Verification items for the finished model (mm, model axes). A direction names the side the tool comes from. Coordinates: 2 decimals unless noted, no trailing zeros. Order: outer loops, then holes, each group sorted by start corner. A loop starts at its lowest first (then second) coordinate and runs counter-clockwise, first axis right, second up. Notation, with made-up numbers: M -39.5,23.5 L -24.5,23.5 A16 ccw -24.5,48.5 Z; hole C 15.25,-26.5 d4. An arc over 180 degrees is marked long. Use one line per item in the form item = value. Start each with the question number.
```python
from build123d import *

# Parameters (mm, degrees)
CUBE002_W     = 38
CUBE002_H     = 3
CUBE002_DEPTH = 43.8
CUBE001_W     = 38
CUBE001_H     = 19
CUBE001_DEPTH = 43.8
SKETCH002_W   = 38
SKETCH002_H   = 43.8
PAD002_DEPTH  = 17
SKETCH003_R   = 1.2
PAD003_DEPTH  = 9
SKETCH004_W   = 38
SKETCH004_H   = 43.8
SKETCH004_W_2 = 34
SKETCH004_H_2 = 39.8
PAD004_DEPTH  = 9


with BuildPart() as cube002:
    # cube002 → cube002 (new body)
    with BuildSketch(Plane(origin=(-19, -3, 0), x_dir=(1, 0, 0), z_dir=(0, 0, 1))):
        with Locations((19, 1.5)):
            Rectangle(CUBE002_W, CUBE002_H)
    extrude(amount=CUBE002_DEPTH)


with BuildPart() as cube001:
    # cube001 → cube001 (new body)
    with BuildSketch(Plane(origin=(-19, 0, 0), x_dir=(1, 0, 0), z_dir=(0, 0, 1))):
        with Locations((19, 9.5)):
            Rectangle(CUBE001_W, CUBE001_H)
    extrude(amount=CUBE001_DEPTH)


with BuildPart() as group003:
    # sphere001 → sphere001 (revolve)
    with BuildSketch(Plane(origin=(0, 0, 24.8), x_dir=(1, 0, 0), z_dir=(0, -1, 0))):
        with BuildLine():
            ThreePointArc((0, -14), (14, 0), (0, 14))
            Line((0, 14), (0, -14))
        make_face()
    revolve(axis=Axis((0, 0, 24.8), (0, 0, 1)))

    # intersection: intersect cube001
    add(cube001.part, mode=Mode.INTERSECT)

    # Group003: union cube002
    add(cube002.part)


with BuildPart() as pad004:
    # Pad002 base: copy of Group003
    add(group003.part)

    # Sketch002 → Pad002 (new body)
    with BuildSketch(Plane.XZ.offset(3)):
        with Locations((0, 21.9)):
            Rectangle(SKETCH002_W, SKETCH002_H)
    extrude(amount=-PAD002_DEPTH)

    # Cut: cut Group003
    add(group003.part, mode=Mode.SUBTRACT)


with BuildPart() as pad004_1:
    # Cut placement: moved
    add(pad004.part.moved(Location((38, -12, -3))))

    # Sketch003 → Pad003 (new body)
    with BuildSketch(Plane(origin=(38, -12, -3), x_dir=(1, 0, 0), z_dir=(0, -1, 0))):
        with Locations((-11.577259, 35.235146)):
            Circle(SKETCH003_R)
        with Locations((10.612975, 13.512618)):
            Circle(SKETCH003_R)
        with Locations((3.638596, 9.535999)):
            Circle(SKETCH003_R)
    extrude(amount=PAD003_DEPTH)

    # Sketch004 → Pad004 (new body)
    with BuildSketch(Plane(origin=(38, -12, -3), x_dir=(1, 0, 0), z_dir=(0, -1, 0))):
        with Locations((0, 21.9)):
            Rectangle(SKETCH004_W, SKETCH004_H)
        with Locations((0, 21.9)):
            Rectangle(SKETCH004_W_2, SKETCH004_H_2, mode=Mode.SUBTRACT)
    extrude(amount=PAD004_DEPTH)


solid = pad004_1.part
```
1. Depth check by flat-ended pin: P1, Ø10, axis at x = 47.5, z = 18.5, coming from the -Y side; P2, Ø6, axis at x = 43.5, z = 16.5, coming from the -Y side; P3, Ø10, axis at x = 35, z = 20.5, coming from the -Y side. Enter the tip coordinate at first touch or a pass-through.
2. Cross-section at C-C on x = 22. Enter the section's corners in (y, z), and give its area (3 significant figures).
3. Cross-section at A-A on y = -13. Enter the section's corners in (x, z), and give its area (3 significant figures).
4. Cross-section at B-B on z = 37. Enter the section's corners in (x, y).
5. Cross-section at D-D on y = -8.75. Enter the section's corners in (x, z), and give its area (3 significant figures).
6. Material ranges on line 1 along Z through (x, y) = (31.5, -17.5); line 2 along X through (y, z) = (-17.75, 33); line 3 along Z through (x, y) = (41, -19.5), recorded low to high.
7. Tool access check on faces 4 (the flat face through (30, -12, 10)), 5 (the flat face through (38, -9, -3)). Record the directions out of +Z, -Z, +X, -X, +Y, -Y that give a thin tool (end or side, any length) a straight path to the whole face; none if there is none.
8. Release check for a two-part mould opening along X. For faces 1 (the flat face through (38, -9, 40.8)), 2 (the cylindrical face through (42.75, -16.44, 6.08)), 3 (the flat face through (19, -9, 19)) record: pulls with the +X half, pulls with the -X half, needs draft (parallel to the pull), parting line crosses it, or undercut.
Final values:
q1.P1 = -12
q1.P2 = -2.9
q1.P3 = -0.7
q2.outline = M -21,-3 L 2,-3 L 2,40.8 L -21,40.8 L -21,38.8 L -12,38.8 L -12,-1 L -21,-1 Z
q2.area = 649 mm2
q3.outline = M 19,-3 L 57,-3 L 57,40.8 L 19,40.8 Z; C 26.42,32.24 d2.4; C 41.64,6.54 d2.4; C 48.61,10.51 d2.4; hole M 21,-1 L 55,-1 L 55,38.8 L 21,38.8 Z
q3.area = 325 mm2
q4.outline = M 19,-21 L 21,-21 L 21,-12 L 55,-12 L 55,-21 L 57,-21 L 57,2 L 19,2 Z
q5.outline = M 19,-3 L 57,-3 L 57,40.8 L 19,40.8 Z; hole C 38,21.8 d27.24
q5.area = 1,080 mm2
q6.line_1 = -3 to -1, 38.8 to 40.8
q6.line_2 = 19 to 21, 25.5 to 27.35, 55 to 57
q6.line_3 = -3 to -1, 5.52 to 7.55, 38.8 to 40.8
q7.face_4 = -Y
q7.face_5 = -Z, +X, -X, +Y, -Y
q8.face_1 = needs draft
q8.face_2 = undercut
q8.face_3 = pulls with the -X half
